```python
from build123d import *

# Parameters (mm, degrees)
BOSS_EXTRUDE1_DEPTH = 5


with BuildPart() as part:
    # Sketch1 → Boss-Extrude1 (new body)
    with BuildSketch(Plane.XY):
        with BuildLine():
            Line((1.5, 3.125), (1.5, -3.125))
            Line((1.5, -3.125), (-1.5, -3.125))
            Line((-1.5, -3.125), (-1.5, 3.125))
            ThreePointArc((-1.5, 3.125), (-2.958039892, -5.675824881), (5, -1.644696007))
            ThreePointArc((5, -1.644696007), (4.031128874, 1.313343884), (1.5, 3.125))
        make_face()
    extrude(amount=BOSS_EXTRUDE1_DEPTH)


solid = part.part
```
Source: CAD feature listing. Evaluate the final solid. Frame: model axes, mm. A direction names the side the tool comes from. Round coordinates to 2 decimals unless told otherwise and drop trailing zeros. Loops run counter-clockwise (first coordinate to the right, second up) from the corner with the lowest first, then second, coordinate; pieces in that order, holes last. Notation, with made-up numbers: M -40,20 L 9,20 A18 cw 9,50 Z; hole C 43,23.25 d9. An arc over 180 degrees is marked long. Use a Markdown table: item, result. Add a question column.
1. Cut plane A-A, the plane y = -1.5. Output: boundary loops of the cut face in (x, z), and give its area (3 significant figures).
2. Set-up query: faces 1 (the flat face through (-1.5, 0, 2)), 2 (the flat face through (0, -4, 0)). Return all of +Z, -Z, +X, -X, +Y, -Y with unobstructed straight access to the full face (end or side cutting, diameter ignored); none if empty.
3. Cut plane C-C, the plane y = -0.5. Output: boundary loops of the cut face in (x, z).
4. Cut plane D-D, the plane x = 0. Output: boundary loops of the cut face in (y, z) (3 decimals), and give its area (3 significant figures).
5. Ray query, line 1 along X through (y, z) = (-2.75, 2.1); line 2 along X through (y, z) = (2.75, 2.3); line 3 along Y through (x, z) = (-0.5, 0.35) (3 decimals). Return the intervals inside material, ascending. Write a range as [from, to].
6. Cut plane B-B, the plane z = 1.85. Output: boundary loops of the cut face in (x, y) (3 decimals), and give its area (3 significant figures).
7. Pull-direction query (X, two-part tool) for faces 3 (the flat face through (0, -3.125, 2)), 4 (the flat face through (0, -4, 5)); classes: +X half, -X half, draft (parallel to the pull), parting line (faces both ways), or undercut.
8. Contact query for flat-ended pins moving along their axis: pin 1 (2.5 mm diameter, centred on y = 0, z = 2, fed in from -X); pin 2 (1 mm diameter, centred on x = 0.5, z = 3, fed in from +Y) (3 decimals); pin 3 (1 mm diameter, centred on y = 0, z = 1.5, fed in from -X). Output: stop coordinate, or through.
Solution:
| question | item | result |
|---|---|---|
| 1 | outline | M -5,0 L -1.5,0 L -1.5,5 L -5,5 Z; M 1.5,0 L 5,0 L 5,5 L 1.5,5 Z |
| 1 | area | 35.0 mm2 |
| 2 | face 1 | +Z, -Z, +Y |
| 2 | face 2 | -Z, +X, -X, +Y, -Y |
| 3 | outline | M -4.87,0 L -1.5,0 L -1.5,5 L -4.87,5 Z; M 1.5,0 L 4.87,0 L 4.87,5 L 1.5,5 Z |
| 4 | outline | M -6.645,0 L -3.125,0 L -3.125,5 L -6.645,5 Z |
| 4 | area | 17.6 mm2 |
| 5 | line 1 | x = [-4.88, -1.5], [1.5, 4.88] |
| 5 | line 2 | x = [-2.38, -1.5], [1.5, 2.38] |
| 5 | line 3 | y = [-6.62, -3.125] |
| 6 | outline | M -1.5,-3.125 L -1.5,3.125 A5 ccw long 1.5,3.125 L 1.5,-3.125 Z |
| 6 | area | 59.3 mm2 |
| 7 | face 3 | undercut |
| 7 | face 4 | draft |
| 8 | pin 1 | stops at x = -4.98 |
| 8 | pin 2 | stops at y = -3.125 |
| 8 | pin 3 | stops at x = -4.87 |
